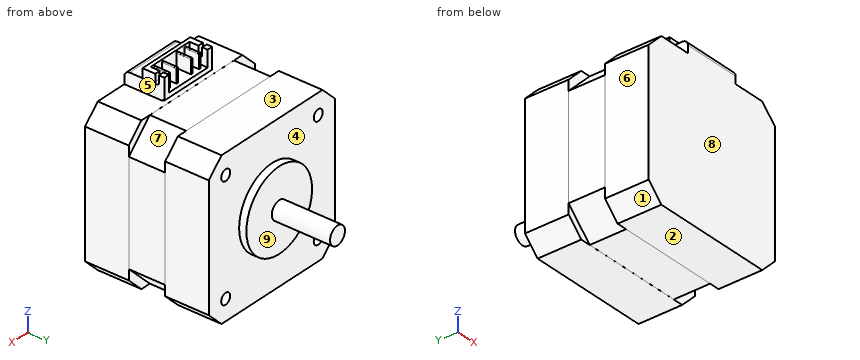
from build123d import *

# Parameters (mm, degrees)
SKETCH1_W               = 42.3
SKETCH1_H               = 42.3
BOSS_EXTRUDE1_DEPTH     = 34
SKETCH2_R               = 11
BOSS_EXTRUDE2_DEPTH     = 2
SKETCH3_R               = 2.5
BOSS_EXTRUDE3_DEPTH     = 16
CUT_EXTRUDE1_DEPTH      = 19
CUT_EXTRUDE1_DEPTH_BACK = 35
SKETCH5_W               = 33.814718626
SKETCH5_H               = 10
CUT_EXTRUDE2_DEPTH      = 0.01
CUT_EXTRUDE3_START      = -12
CUT_EXTRUDE3_DEPTH      = 10
CIRPATTERN1_COUNT       = 4
SKETCH7_R               = 1.5
CUT_EXTRUDE4_DEPTH      = 4.5
SKETCH8_W               = 16
SKETCH8_H               = 11
BOSS_EXTRUDE4_DEPTH     = 6
SKETCH9_W               = 16
SKETCH9_H               = 5
CUT_EXTRUDE5_DEPTH      = 2.5
FILLET1_R               = 1.5
SKETCH10_W              = 13
SKETCH10_H              = 4.5
CUT_EXTRUDE6_DEPTH      = 5
CUT_EXTRUDE7_DEPTH      = 30.15
BOSS_EXTRUDE5_DEPTH     = 4
SKETCH13_W              = 16
SKETCH13_H              = 0.25
CUT_EXTRUDE8_DEPTH      = 0.5
FILLET2_R               = 0.125


with BuildPart() as part:
    # Sketch1 → Boss-Extrude1 (new body)
    with BuildSketch(Plane(origin=(0, 0, 0), x_dir=(1, 0, 0), z_dir=(0, 1, 0))):
        Rectangle(SKETCH1_W, SKETCH1_H)
    extrude(amount=BOSS_EXTRUDE1_DEPTH)

    # Sketch2 → Boss-Extrude2 (add)
    with BuildSketch(Plane(origin=(0, 34, 0), x_dir=(1, 0, 0), z_dir=(0, 1, 0))):
        Circle(SKETCH2_R)
    extrude(amount=BOSS_EXTRUDE2_DEPTH)

    # Sketch3 → Boss-Extrude3 (add)
    with BuildSketch(Plane(origin=(0, 36, 0), x_dir=(1, 0, 0), z_dir=(0, 1, 0))):
        Circle(SKETCH3_R)
    extrude(amount=BOSS_EXTRUDE3_DEPTH)

    # Sketch4 → Cut-Extrude1 (cut, two sides)
    with BuildSketch(Plane(origin=(0, 34, 0), x_dir=(1, 0, 0), z_dir=(0, 1, 0))) as cut_extrude1_sk:
        Polygon((-21.15, 16.907359313), (-16.907359313, 21.15), (-21.15, 21.15), align=None)
        Polygon((21.15, 21.15), (21.15, 16.907359313), (16.907359313, 21.15), align=None)
        Polygon((21.15, -16.907359313), (16.907359313, -21.15), (21.15, -21.15), align=None)
        Polygon((-21.15, -21.15), (-21.15, -16.907359313), (-16.907359313, -21.15), align=None)
    extrude(amount=CUT_EXTRUDE1_DEPTH, mode=Mode.SUBTRACT)
    extrude(cut_extrude1_sk.sketch, amount=-CUT_EXTRUDE1_DEPTH_BACK, mode=Mode.SUBTRACT)

    # Sketch5 → Cut-Extrude2 (cut)
    with BuildSketch(Plane(origin=(21.15, 0, 0), x_dir=(0, 0, -1), z_dir=(1, 0, 0))):
        with Locations((0, 17)):
            Rectangle(SKETCH5_W, SKETCH5_H)
    cut_extrude2 = extrude(amount=-CUT_EXTRUDE2_DEPTH, mode=Mode.SUBTRACT)

    # Sketch6 → Cut-Extrude3 (cut)
    with BuildSketch(Plane(origin=(0, 34, 0), x_dir=(1, 0, 0), z_dir=(0, 1, 0)).offset(CUT_EXTRUDE3_START)):
        Polygon((21.15, 14.078932188), (14.078932188, 21.15), (21.15, 21.15), align=None)
    cut_extrude3 = extrude(amount=-CUT_EXTRUDE3_DEPTH, mode=Mode.SUBTRACT)

    # CirPattern1: Cut-Extrude2, Cut-Extrude3 ×4 about axis
    cirpattern1_axis = Axis((0, 0, 0), (0, 1, 0))
    for i in range(1, CIRPATTERN1_COUNT):
        add(cut_extrude2.rotate(cirpattern1_axis, i * 360 / CIRPATTERN1_COUNT), mode=Mode.SUBTRACT)
        add(cut_extrude3.rotate(cirpattern1_axis, i * 360 / CIRPATTERN1_COUNT), mode=Mode.SUBTRACT)

    # Sketch7 → Cut-Extrude4 (cut)
    with BuildSketch(Plane(origin=(0, 34, 0), x_dir=(1, 0, 0), z_dir=(0, 1, 0))):
        with Locations((15.5, 15.5)):
            Circle(SKETCH7_R)
        with Locations((15.5, -15.5)):
            Circle(SKETCH7_R)
        with Locations((-15.5, -15.5)):
            Circle(SKETCH7_R)
        with Locations((-15.5, 15.5)):
            Circle(SKETCH7_R)
    extrude(amount=-CUT_EXTRUDE4_DEPTH, mode=Mode.SUBTRACT)

    # Sketch8 → Boss-Extrude4 (add)
    with BuildSketch(Plane.XY.offset(21.15)):
        with Locations((0, 5.5)):
            Rectangle(SKETCH8_W, SKETCH8_H)
    extrude(amount=BOSS_EXTRUDE4_DEPTH)

    # Sketch9 → Cut-Extrude5 (cut)
    with BuildSketch(Plane.XY.offset(27.15)):
        with Locations((0, 2.5)):
            Rectangle(SKETCH9_W, SKETCH9_H)
    extrude(amount=-CUT_EXTRUDE5_DEPTH, mode=Mode.SUBTRACT)

    # Fillet1
    fillet1_edges = [part.edges().sort_by_distance(p)[0] for p in [
        (0, 0, 24.65),
    ]]
    fillet(fillet1_edges, radius=FILLET1_R)

    # Sketch10 → Cut-Extrude6 (cut)
    with BuildSketch(Plane(origin=(0, 11, 0), x_dir=(1, 0, 0), z_dir=(0, 1, 0))):
        with Locations((0, -24.9)):
            Rectangle(SKETCH10_W, SKETCH10_H)
    extrude(amount=-CUT_EXTRUDE6_DEPTH, mode=Mode.SUBTRACT)

    # Sketch11 → Cut-Extrude7 (cut, through all)
    with BuildSketch(Plane(origin=(8, 0, 0), x_dir=(0, 0, -1), z_dir=(1, 0, 0))):
        with BuildLine():
            Line((-27.15, 9.5), (-25.15, 9.5))
            ThreePointArc((-25.15, 9.5), (-24.65, 9), (-25.15, 8.5))
            Line((-25.15, 8.5), (-27.15, 8.5))
            Line((-27.15, 8.5), (-27.15, 9.5))
        make_face()
    extrude(amount=-CUT_EXTRUDE7_DEPTH, mode=Mode.SUBTRACT)

    # Sketch12 → Boss-Extrude5 (add)
    with BuildSketch(Plane(origin=(0, 6, 0), x_dir=(1, 0, 0), z_dir=(0, 1, 0))):
        with BuildLine():
            Line((-2.667, -22.65), (-2.167, -22.65))
            Line((-2.167, -22.65), (-2.167, -26.4))
            ThreePointArc((-2.167, -26.4), (-2.417, -26.65), (-2.667, -26.4))
            Line((-2.667, -26.4), (-2.667, -22.65))
        make_face()
        with BuildLine():
            Line((5.334, -22.65), (5.334, -26.4))
            ThreePointArc((5.334, -26.4), (5.084, -26.65), (4.834, -26.4))
            Line((4.834, -26.4), (4.834, -22.65))
            Line((4.834, -22.65), (5.334, -22.65))
        make_face()
        with BuildLine():
            Line((-4.834, -22.65), (-5.334, -22.65))
            Line((-5.334, -22.65), (-5.334, -26.4))
            ThreePointArc((-5.334, -26.4), (-5.084, -26.65), (-4.834, -26.4))
            Line((-4.834, -26.4), (-4.834, -22.65))
        make_face()
        with BuildLine():
            Line((2.167, -22.65), (2.167, -26.4))
            ThreePointArc((2.167, -26.4), (2.417, -26.65), (2.667, -26.4))
            Line((2.667, -26.4), (2.667, -22.65))
            Line((2.667, -22.65), (2.167, -22.65))
        make_face()
    extrude(amount=BOSS_EXTRUDE5_DEPTH)

    # Sketch13 → Cut-Extrude8 (cut)
    with BuildSketch(Plane(origin=(0, 11, 0), x_dir=(1, 0, 0), z_dir=(0, 1, 0))):
        with Locations((0, -21.275)):
            Rectangle(SKETCH13_W, SKETCH13_H)
    extrude(amount=-CUT_EXTRUDE8_DEPTH, mode=Mode.SUBTRACT)

    # Fillet2
    fillet2_edges = [part.edges().sort_by_distance(p)[0] for p in [
        (0, 10.5, 21.4),
    ]]
    fillet(fillet2_edges, radius=FILLET2_R)


solid = part.part
Build history of the part. All positions in model axes, mm. Face numbers are marked on the shaded views. A direction names the side the tool comes from. Give positions to 0.01 mm unless a question says otherwise; leave off trailing zeros. Write each loop counter-clockwise with the first axis right and the second up, starting at its lowest first coordinate (ties: lowest second). Pieces come first, ordered by that corner, then holes. Notation, with made-up numbers: (-24, 57) - (-9, 57) arc R19 ccw to (-9, 66) - close; hole circle Ø8 at (-31, -0.75). An arc over 180 degrees is marked (long way). Use one line per item in the form item = value. Start each with the question number.
1. Band-saw the part on D-D on x = -18. Write the cut outline in (y, z).
2. Drop flat-ended pins along their axis: pin 1 Ø0.8 at (x, z) = (7.5, 26) entering from -Y; pin 2 Ø1.5 at (x, z) = (15.5, 15) entering from +Y; pin 3 Ø1 at (y, z) = (5.5, 21.5) entering from -X. Give the stop position or say it passes through.
3. Probe line 1 (X direction, y = 32.35, z = 15.5); line 2 (X direction, y = 32, z = 15). List the from-to ranges inside material, lowest first. Write a range as [from, to].
4. Band-saw the part on C-C on y = 17.5. Write the cut outline in (x, z).
5. 3-axis set-ups, long thin cutter, end or side, ignore diameter. For the marked faces 1, 2, 3, 4 and 5: which of +Z, -Z, +X, -X, +Y, -Y reach the whole face in a straight line?
6. Two-plate mould, pull along Y, no slides. Class the marked faces 6, 7, 8 and 9: released by +Y, released by -Y, zero draft, split by the parting line, or undercut.
Conclusion:
q1.outline = (0, -20.06) - (12, -20.06) - (12, -17.23) - (22, -17.23) - (22, -20.06) - (34, -20.06) - (34, 20.06) - (22, 20.06) - (22, 17.23) - (12, 17.23) - (12, 20.06) - (0, 20.06) - close
q2.pin_1 = 5
q2.pin_2 = 29.5
q2.pin_3 = -17.06
q3.line_1 = [-21.15, -17], [-14, 14], [17, 21.15]
q3.line_2 = [-21.15, -16.91], [-14.09, 14.09], [16.91, 21.15]
q4.outline = (-21.14, -14.09) - (-14.09, -21.14) - (14.09, -21.14) - (21.14, -14.09) - (21.14, 14.09) - (14.09, 21.14) - (-14.09, 21.14) - (-21.14, 14.09) - close
q5.face_1 = -Z, -X, +Y, -Y
q5.face_2 = -Z, +X, -X, +Y, -Y
q5.face_3 = +Z, +X, -X, +Y
q5.face_4 = +Y
q5.face_5 = +Z, +X, +Y, -Y
q6.face_6 = zero draft
q6.face_7 = undercut
q6.face_8 = released by -Y
q6.face_9 = released by +Y
